Check sheet for the drawn part. Datum: minimum x, y, z corner. Units: mm. A direction names the side the tool comes from. Round coordinates to 2 decimals unless told otherwise and drop trailing zeros. Write each loop counter-clockwise with the first axis right and the second up, starting at its lowest first coordinate (ties: lowest second). Pieces come first, ordered by that corner, then holes. Notation, with made-up numbers: (56.5, -31.5) - (73.5, -31.5) arc R29 ccw to (73.5, -11.5) - close; hole circle Ø5 at (-26.75, 71.5). An arc over 180 degrees is marked (long way). Write each question's results on one line, items separated by ' | '.
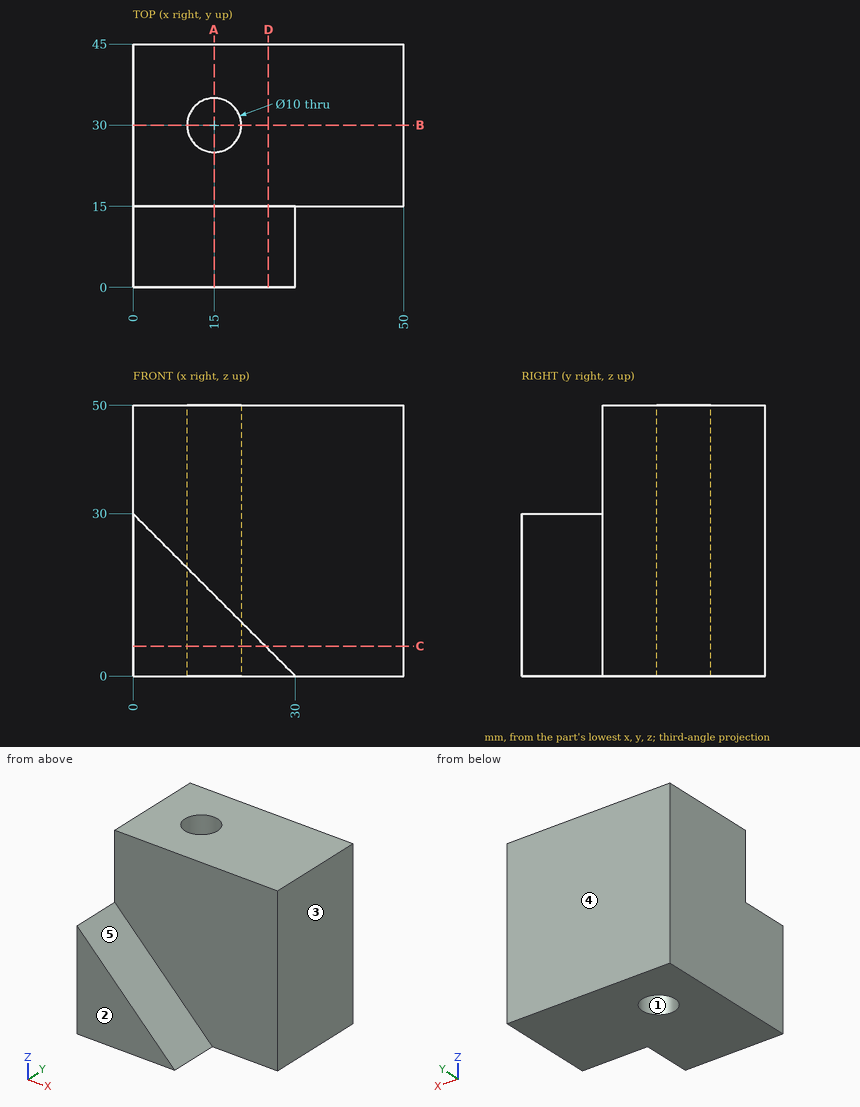
(1) Section check A-A (x = 15). Record the cut outline in (y, z).
Answer:
outline: (0, 0) - (25, 0) - (25, 50) - (15, 50) - (15, 15) - (0, 15) - close; (35, 0) - (45, 0) - (45, 50) - (35, 50) - close
(2) Go/stop test with flat-tipped pins: pin 1 Ø12 at (x, y) = (27, 18) entering from -Z; pin 2 Ø12 at (x, z) = (35, 19) entering from -Y. Record where each tip stops, or that it passes through.
Answer:
pin 1: z = 0 | pin 2: y = 15
(3) Mould release check, pull along X, two halves, no side actions. Record for the marked faces 1, 2 and 3: released by +X, released by -X, zero draft, split by the parting line, or undercut.
Answer:
face 1: undercut | face 2: zero draft | face 3: released by +X
(4) Set-up check for the marked faces 4 and 5: record each of +Z, -Z, +X, -X, +Y, -Y from which the full face is reachable in a straight line by a thin tool's end or side.
Answer:
face 4: +Z, -Z, +X, -X, +Y | face 5: +Z, +X, -Y
(5) Thickness scan on L1, parallel to Y at x = 15, z = 35; L2, parallel to Y at x = 35.5, z = 42.5; L3, parallel to X at y = 6, z = 10. Record the ranges inside material, lowest first.
Answer:
L1: 15 to 25, 35 to 45 | L2: 15 to 45 | L3: 0 to 20
(6) Section check B-B (y = 30). Record the cut outline in (x, z), plus the area to 3 significant figures.
Answer:
outline: (0, 0) - (10, 0) - (10, 50) - (0, 50) - close; (20, 0) - (50, 0) - (50, 50) - (20, 50) - close | area: 2,000 mm2
(7) Section check D-D (x = 25). Record the cut outline in (y, z).
Answer:
outline: (0, 0) - (45, 0) - (45, 50) - (15, 50) - (15, 5) - (0, 5) - close
(8) Section check C-C (z = 5.5). Record the cut outline in (x, y), plus the area to 3 significant figures.
Answer:
outline: (0, 0) - (24.5, 0) - (24.5, 15) - (50, 15) - (50, 45) - (0, 45) - close; hole circle Ø10 at (15, 30) | area: 1,790 mm2
